The listing builds one solid part. Answer for the finished solid, in the listing's coordinates (mm). A direction names the side the tool comes from. Give positions to 0.01 mm unless a question says otherwise; leave off trailing zeros. Write each loop counter-clockwise with the first axis right and the second up, starting at its lowest first coordinate (ties: lowest second). Pieces come first, ordered by that corner, then holes. Notation, with made-up numbers: (61.25, -17) -> (93.25, -17) arc R27 ccw to (93.25, 5) -> close; hole circle Ø3 at (36, -38). An arc over 180 degrees is marked (long way). One line per question, with ' | ' between items.
from build123d import *

# Parameters (mm, degrees)
SKETCH_1_W          = 100
SKETCH_1_H          = 75
SKETCH_1_R          = 3.3
EXTRUDE_1_DEPTH     = 6
EXTRUDE_2_DEPTH     = 40
CUT_EXTRUDE_1_REACH = 102.093
SKETCH_3_R          = 1.5
SKETCH_3_W          = 35
SKETCH_3_H          = 29.2
FILLET_1_R          = 6
FILLET_2_R          = 5


with BuildPart() as part:
    # 스케치1 → 보스-돌출1 (new body)
    with BuildSketch(Plane.XY):
        Rectangle(SKETCH_1_W, SKETCH_1_H)
        with Locations((-37.5, 25)):
            Circle(SKETCH_1_R, mode=Mode.SUBTRACT)
        with Locations((37.5, 25)):
            Circle(SKETCH_1_R, mode=Mode.SUBTRACT)
        with Locations((37.5, -25)):
            Circle(SKETCH_1_R, mode=Mode.SUBTRACT)
        with Locations((-37.5, -25)):
            Circle(SKETCH_1_R, mode=Mode.SUBTRACT)
    extrude(amount=EXTRUDE_1_DEPTH)

    # 스케치2 → 보스-돌출2 (add)
    with BuildSketch(Plane.XY.offset(6)):
        Polygon((-18.6, 20.7), (-18.6, 28.7), (-30.6, 28.7), (-30.6, -28.7), (-18.6, -28.7), (-18.6, -20.7), (-26.6, -20.7), (-26.6, 20.7), align=None)
        Polygon((8.6, -20.7), (0.6, -20.7), (0.6, -28.7), (12.6, -28.7), (12.6, 28.7), (0.6, 28.7), (0.6, 20.7), (8.6, 20.7), align=None)
    extrude(amount=EXTRUDE_2_DEPTH)

    # 컷-돌출1: up to this face of the body (flat: up to its plane)
    cut_extrude_1_end = Plane(part.part.faces().sort_by_distance((12.6, 0, 26))[0])
    # 스케치3 → 컷-돌출1 (cut, up to the picked face)
    with BuildSketch(Plane.ZY.offset(30.6), mode=Mode.PRIVATE) as cut_extrude_1_sk1:
        with Locations((8.8, 11)):
            Circle(SKETCH_3_R)
    cut_extrude_1_tool1 = split(extrude(cut_extrude_1_sk1.sketch, amount=-CUT_EXTRUDE_1_REACH, mode=Mode.PRIVATE), bisect_by=cut_extrude_1_end, keep=Keep.BOTH, mode=Mode.PRIVATE)
    # 스케치3 → 컷-돌출1 (cut, up to the picked face)
    with BuildSketch(Plane.ZY.offset(30.6), mode=Mode.PRIVATE) as cut_extrude_1_sk2:
        with Locations((14.1, 17.3)):
            Circle(SKETCH_3_R)
    cut_extrude_1_tool2 = split(extrude(cut_extrude_1_sk2.sketch, amount=-CUT_EXTRUDE_1_REACH, mode=Mode.PRIVATE), bisect_by=cut_extrude_1_end, keep=Keep.BOTH, mode=Mode.PRIVATE)
    # 스케치3 → 컷-돌출1 (cut, up to the picked face)
    with BuildSketch(Plane.ZY.offset(30.6), mode=Mode.PRIVATE) as cut_extrude_1_sk3:
        with Locations((36.1, 17.3)):
            Circle(SKETCH_3_R)
    cut_extrude_1_tool3 = split(extrude(cut_extrude_1_sk3.sketch, amount=-CUT_EXTRUDE_1_REACH, mode=Mode.PRIVATE), bisect_by=cut_extrude_1_end, keep=Keep.BOTH, mode=Mode.PRIVATE)
    # 스케치3 → 컷-돌출1 (cut, up to the picked face)
    with BuildSketch(Plane.ZY.offset(30.6), mode=Mode.PRIVATE) as cut_extrude_1_sk4:
        with Locations((8.8, -11)):
            Circle(SKETCH_3_R)
    cut_extrude_1_tool4 = split(extrude(cut_extrude_1_sk4.sketch, amount=-CUT_EXTRUDE_1_REACH, mode=Mode.PRIVATE), bisect_by=cut_extrude_1_end, keep=Keep.BOTH, mode=Mode.PRIVATE)
    # 스케치3 → 컷-돌출1 (cut, up to the picked face)
    with BuildSketch(Plane.ZY.offset(30.6), mode=Mode.PRIVATE) as cut_extrude_1_sk5:
        with Locations((14.1, -17.3)):
            Circle(SKETCH_3_R)
    cut_extrude_1_tool5 = split(extrude(cut_extrude_1_sk5.sketch, amount=-CUT_EXTRUDE_1_REACH, mode=Mode.PRIVATE), bisect_by=cut_extrude_1_end, keep=Keep.BOTH, mode=Mode.PRIVATE)
    # 스케치3 → 컷-돌출1 (cut, up to the picked face)
    with BuildSketch(Plane.ZY.offset(30.6), mode=Mode.PRIVATE) as cut_extrude_1_sk6:
        with Locations((36.1, -17.3)):
            Circle(SKETCH_3_R)
    cut_extrude_1_tool6 = split(extrude(cut_extrude_1_sk6.sketch, amount=-CUT_EXTRUDE_1_REACH, mode=Mode.PRIVATE), bisect_by=cut_extrude_1_end, keep=Keep.BOTH, mode=Mode.PRIVATE)
    # 스케치3 → 컷-돌출1 (cut, up to the picked face)
    with BuildSketch(Plane.ZY.offset(30.6), mode=Mode.PRIVATE) as cut_extrude_1_sk7:
        with Locations((28.5, 0)):
            Rectangle(SKETCH_3_W, SKETCH_3_H)
    cut_extrude_1_tool7 = split(extrude(cut_extrude_1_sk7.sketch, amount=-CUT_EXTRUDE_1_REACH, mode=Mode.PRIVATE), bisect_by=cut_extrude_1_end, keep=Keep.BOTH, mode=Mode.PRIVATE)
    add(cut_extrude_1_tool1.solids().sort_by(Axis((-30.6, 11, 8.8), (1, 0, 0)))[0], mode=Mode.SUBTRACT)
    add(cut_extrude_1_tool2.solids().sort_by(Axis((-30.6, 17.3, 14.1), (1, 0, 0)))[0], mode=Mode.SUBTRACT)
    add(cut_extrude_1_tool3.solids().sort_by(Axis((-30.6, 17.3, 36.1), (1, 0, 0)))[0], mode=Mode.SUBTRACT)
    add(cut_extrude_1_tool4.solids().sort_by(Axis((-30.6, -11, 8.8), (1, 0, 0)))[0], mode=Mode.SUBTRACT)
    add(cut_extrude_1_tool5.solids().sort_by(Axis((-30.6, -17.3, 14.1), (1, 0, 0)))[0], mode=Mode.SUBTRACT)
    add(cut_extrude_1_tool6.solids().sort_by(Axis((-30.6, -17.3, 36.1), (1, 0, 0)))[0], mode=Mode.SUBTRACT)
    add(cut_extrude_1_tool7.solids().sort_by(Axis((-30.6, 0, 28.5), (1, 0, 0)))[0], mode=Mode.SUBTRACT)

    # 필렛1
    fillet_1_edges = [part.edges().sort_by_distance(p)[0] for p in [
        (-18.6, 24.7, 6),
        (-24.6, 28.7, 6),
        (-24.6, -28.7, 6),
        (-18.6, -24.7, 6),
        (0.6, -24.7, 6),
        (6.6, -28.7, 6),
        (6.6, 28.7, 6),
        (0.6, 24.7, 6),
    ]]
    fillet(fillet_1_edges, radius=FILLET_1_R)

    # 필렛2
    # the kernel refuses this fillet: 5 mm, written as the material it takes off along each edge
    with BuildSketch(Plane(origin=(-30.6, 34.7, 12), x_dir=(0, 0.8710924829717933, 0.49111901420127907), z_dir=(0, -0.49111901420127907, 0.8710924829717933))) as fillet_2_piece_1_section:
        with BuildLine():
            CenterArc((6 + FILLET_2_R, -FILLET_2_R), FILLET_2_R, 90, 90)
            Line((6, -FILLET_2_R), (6, 0))
            Line((6, 0), (6 + FILLET_2_R, 0))
        make_face()
    fillet_2_piece_1 = revolve(axis=Axis((-30.6, 34.7, 12), (-1, 0, 0)), revolution_arc=209.414157698, mode=Mode.PRIVATE)
    fillet_2_piece_1 = split(fillet_2_piece_1, bisect_by=Plane(origin=(-29.099532235, 30.223820848, 6), z_dir=(0, 0, 1)), keep=Keep.TOP, mode=Mode.PRIVATE)
    add(fillet_2_piece_1, mode=Mode.SUBTRACT)
    with BuildSketch(Plane(origin=(12.6, 34.7, 12), x_dir=(0, 0.8710924829717934, 0.4911190142012785), z_dir=(0, -0.4911190142012785, 0.8710924829717934))) as fillet_2_piece_2_section:
        with BuildLine():
            CenterArc((6 + FILLET_2_R, FILLET_2_R), FILLET_2_R, 180, 90)
            Line((6 + FILLET_2_R, 0), (6, 0))
            Line((6, 0), (6, FILLET_2_R))
        make_face()
    fillet_2_piece_2 = revolve(axis=Axis((12.6, 34.7, 12), (-1, 0, 0)), revolution_arc=209.414157698, mode=Mode.PRIVATE)
    fillet_2_piece_2 = split(fillet_2_piece_2, bisect_by=Plane(origin=(11.099532075, 30.223821009, 6), z_dir=(0, 0, 1)), keep=Keep.TOP, mode=Mode.PRIVATE)
    add(fillet_2_piece_2, mode=Mode.SUBTRACT)
    with BuildSketch(Plane(origin=(12.6, -34.7, 12), x_dir=(0, -0.8710924829717933, 0.49111901420127907), z_dir=(0, 0.49111901420127907, 0.8710924829717933))) as fillet_2_piece_3_section:
        with BuildLine():
            CenterArc((6 + FILLET_2_R, -FILLET_2_R), FILLET_2_R, 90, 90)
            Line((6, -FILLET_2_R), (6, 0))
            Line((6, 0), (6 + FILLET_2_R, 0))
        make_face()
    fillet_2_piece_3 = revolve(axis=Axis((12.6, -34.7, 12), (1, 0, 0)), revolution_arc=209.414157698, mode=Mode.PRIVATE)
    fillet_2_piece_3 = split(fillet_2_piece_3, bisect_by=Plane(origin=(11.099532513, -30.223820921, 6), z_dir=(0, 0, 1)), keep=Keep.TOP, mode=Mode.PRIVATE)
    add(fillet_2_piece_3, mode=Mode.SUBTRACT)
    with BuildSketch(Plane(origin=(-30.6, -34.7, 12), x_dir=(0, -0.8710924829717931, 0.4911190142012795), z_dir=(0, 0.4911190142012795, 0.8710924829717931))) as fillet_2_piece_4_section:
        with BuildLine():
            CenterArc((6 + FILLET_2_R, FILLET_2_R), FILLET_2_R, 180, 90)
            Line((6 + FILLET_2_R, 0), (6, 0))
            Line((6, 0), (6, FILLET_2_R))
        make_face()
    fillet_2_piece_4 = revolve(axis=Axis((-30.6, -34.7, 12), (1, 0, 0)), revolution_arc=209.414157698, mode=Mode.PRIVATE)
    fillet_2_piece_4 = split(fillet_2_piece_4, bisect_by=Plane(origin=(-29.099532146, -30.223820899, 6), z_dir=(0, 0, 1)), keep=Keep.TOP, mode=Mode.PRIVATE)
    add(fillet_2_piece_4, mode=Mode.SUBTRACT)
    with BuildSketch(Plane(origin=(-30.6, 28.7, 12), x_dir=(1, 0, 0), z_dir=(0, 0, 1)), Plane(origin=(12.6, -28.7, 12), x_dir=(-1, 0, 0), z_dir=(0, 0, 1))) as fillet_2_piece_5:
        with BuildLine():
            CenterArc((FILLET_2_R, -FILLET_2_R), FILLET_2_R, 90, 90)
            Line((0, -FILLET_2_R), (0, 0))
            Line((0, 0), (FILLET_2_R, 0))
        make_face()
    extrude(amount=46.5, mode=Mode.SUBTRACT)
    with BuildSketch(Plane(origin=(-30.6, -28.7, 12), x_dir=(1, 0, 0), z_dir=(0, 0, 1)), Plane(origin=(12.6, 28.7, 12), x_dir=(-1, 0, 0), z_dir=(0, 0, 1))) as fillet_2_piece_6:
        with BuildLine():
            CenterArc((FILLET_2_R, FILLET_2_R), FILLET_2_R, 180, 90)
            Line((0, FILLET_2_R), (0, 0))
            Line((0, 0), (FILLET_2_R, 0))
        make_face()
    extrude(amount=46.5, mode=Mode.SUBTRACT)


solid = part.part
Item 1: Find section B-B (y = 17.3). Write down the section's boundary in (x, z), then the cut area to 3 significant figures.
Answers below:
outline: (-50, 0) -> (50, 0) -> (50, 6) -> (12.6, 6) -> (12.6, 12.6) -> (8.6, 12.6) -> (8.6, 6) -> (-26.6, 6) -> (-26.6, 12.6) -> (-30.6, 12.6) -> (-30.6, 6) -> (-50, 6) -> close; (-30.6, 15.6) -> (-26.6, 15.6) -> (-26.6, 34.6) -> (-30.6, 34.6) -> close; (-30.6, 37.6) -> (-26.6, 37.6) -> (-26.6, 46) -> (-30.6, 46) -> close; (8.6, 15.6) -> (12.6, 15.6) -> (12.6, 34.6) -> (8.6, 34.6) -> close; (8.6, 37.6) -> (12.6, 37.6) -> (12.6, 46) -> (8.6, 46) -> close | area: 872 mm²
Item 2: A tool of negligible diameter and unlimited length cuts with its end or side. For faces 1 (the face through (4, 28.7, 29)), 2 (the face through (-29, 14.6, 28)), 3 (the face through (-29.1, 27.27, 28.76)), 4 (the face through (-29.17, -27.2, 28.76)), 5 (the face through (-16.796, -26.046, 7.711)), from which of +Z, -Z, +X, -X, +Y, -Y can it reach the whole face along a straight path? Write none if from no direction.
Answers below:
face 1: +Z, +X, -X, +Y | face 2: +Z, +X, -X | face 3: +Z, -X, +Y | face 4: +Z, -X, -Y | face 5: +Z, +Y, -Y
Item 3: Consider line 1 (Y direction, x = -37.5, z = 1.95); line 2 (Y direction, x = -29, z = 36); line 3 (X direction, y = 24, z = 44.5). Determine where each line is inside the solid, lowest interval first. Write a range as [from, to].
Answers below:
line 1: [-37.5, -28.3], [-21.7, 21.7], [28.3, 37.5] | line 2: [-27.37, -18.8], [-15.8, -14.6], [14.6, 15.8], [18.8, 27.37] | line 3: [-30.59, -18.6], [0.6, 12.59]
Item 4: Find section A-A (z = 22). Write down the section's boundary in (x, y), then the cut area to 3 significant figures.
Answers below:
outline: (-30.6, -23.7) arc R5 ccw to (-25.6, -28.7) -> (-18.6, -28.7) -> (-18.6, -20.7) -> (-26.6, -20.7) -> (-26.6, -14.6) -> (-30.6, -14.6) -> close; (-30.6, 14.6) -> (-26.6, 14.6) -> (-26.6, 20.7) -> (-18.6, 20.7) -> (-18.6, 28.7) -> (-25.6, 28.7) arc R5 ccw to (-30.6, 23.7) -> close; (0.6, -28.7) -> (7.6, -28.7) arc R5 ccw to (12.6, -23.7) -> (12.6, -14.6) -> (8.6, -14.6) -> (8.6, -20.7) -> (0.6, -20.7) -> close; (0.6, 20.7) -> (8.6, 20.7) -> (8.6, 14.6) -> (12.6, 14.6) -> (12.6, 23.7) arc R5 ccw to (7.6, 28.7) -> (0.6, 28.7) -> close | area: 460 mm²
Item 5: Flat-ended cylindrical pins translate along their axes: pin 1 (5 mm diameter, centred on x = -32, y = 2.5, fed in from +Z); pin 2 (3.5 mm diameter, centred on x = 6, z = 27.5, fed in from +Y); pin 3 (6 mm diameter, centred on x = -33, z = 40.5, fed in from -Y); pin 4 (6 mm diameter, centred on x = -3, z = 40, fed in from -Y). Find the tip coordinate at first contact, or state that the pin passes through.
Answers below:
pin 1: z = 11 | pin 2: y = 28.7 | pin 3: y = -26.07 | pin 4: through
Item 6: Determine the mould class of faces 6 (the face through (10.572, 15.836, 13.775)), 7 (the face through (12.6, 0, 8)), 8 (the face through (34.881, -27.008, 2.958)), 9 (the face through (-40.119, 22.992, 2.958)) for opening direction X: pulls with the +X half, pulls with the -X half, needs draft (parallel to the pull), parting line crosses it, or undercut.
Answers below:
face 6: needs draft | face 7: pulls with the +X half | face 8: undercut | face 9: undercut
Item 7: Find section D-D (x = 37.5). Write down the section's boundary in (y, z), then the cut area to 3 significant figures.
Answers below:
outline: (-37.5, 0) -> (-28.3, 0) -> (-28.3, 6) -> (-37.5, 6) -> close; (-21.7, 0) -> (21.7, 0) -> (21.7, 6) -> (-21.7, 6) -> close; (28.3, 0) -> (37.5, 0) -> (37.5, 6) -> (28.3, 6) -> close | area: 371 mm²
Item 8: Find section C-C (x = -20). Write down the section's boundary in (y, z).
Answers below:
outline: (-37.5, 0) -> (37.5, 0) -> (37.5, 6) -> (34.7, 6) arc R6 cw to (28.7, 12) -> (28.7, 46) -> (20.7, 46) -> (20.7, 6) -> (-20.7, 6) -> (-20.7, 46) -> (-28.7, 46) -> (-28.7, 12) arc R6 cw to (-34.7, 6) -> (-37.5, 6) -> close
